```python
from build123d import *

# Parameters (mm, degrees)
SALIENTE_EXTRUIR1_DEPTH = 15
CROQUIS2_R              = 2.5
CORTAR_EXTRUIR1_DEPTH   = 3.5
CORTAR_EXTRUIR2_START   = -3.5
CROQUIS3_R              = 2.5
CORTAR_EXTRUIR2_DEPTH   = 3.5
CROQUIS4_R              = 2.5
CORTAR_EXTRUIR3_DEPTH   = 2
REDONDEO1_R             = 0.1
CROQUIS5_R              = 1.5
CORTAR_EXTRUIR4_DEPTH   = 26.421447638


with BuildPart() as part:
    # Croquis1 → Saliente-Extruir1 (new body)
    with BuildSketch(Plane.XY):
        with BuildLine():
            Line((-1.5, 11), (1.5, 11))
            ThreePointArc((1.5, 11), (4.328427125, 9.828427125), (5.5, 7))
            Line((5.5, 7), (5.5, -6))
            Line((5.5, -6), (11.5, -6))
            Line((11.5, -6), (11.5, -11))
            Line((11.5, -11), (5.5, -11))
            Line((5.5, -11), (-5.5, -11))
            Line((-5.5, -11), (-11.5, -11))
            Line((-11.5, -11), (-11.5, -6))
            Line((-11.5, -6), (-5.5, -6))
            Line((-5.5, -6), (-5.5, 7))
            ThreePointArc((-5.5, 7), (-4.328427125, 9.828427125), (-1.5, 11))
        make_face()
    extrude(amount=-SALIENTE_EXTRUIR1_DEPTH)

    # Croquis2 → Cortar-Extruir1 (cut)
    with BuildSketch(Plane(origin=(5.5, 0, 0), x_dir=(0, 0, -1), z_dir=(1, 0, 0))):
        with Locations(Location((7.5, 2.7, 0), (0, 0, 90))):
            Circle(CROQUIS2_R)
    extrude(amount=-CORTAR_EXTRUIR1_DEPTH, mode=Mode.SUBTRACT)

    # Croquis3 → Cortar-Extruir2 (cut)
    with BuildSketch(Plane.ZY.offset(5.5).offset(CORTAR_EXTRUIR2_START)):
        with Locations(Location((-7.5, 2.7, 0), (0, 0, 90))):
            Circle(CROQUIS3_R)
    extrude(amount=CORTAR_EXTRUIR2_DEPTH, mode=Mode.SUBTRACT)

    # Croquis4 → Cortar-Extruir3 (cut)
    with BuildSketch(Plane(origin=(0, -6, 0), x_dir=(1, 0, 0), z_dir=(0, 1, 0))):
        with Locations(Location((-8.5, 11, 0), (0, 0, 180))):
            Circle(CROQUIS4_R)
        with Locations(Location((-8.5, 4, 0), (0, 0, 180))):
            Circle(CROQUIS4_R)
        with Locations((8.5, 4)):
            Circle(CROQUIS4_R)
        with Locations((8.5, 11)):
            Circle(CROQUIS4_R)
    extrude(amount=-CORTAR_EXTRUIR3_DEPTH, mode=Mode.SUBTRACT)

    # Redondeo1
    redondeo1_edges = [part.edges().sort_by_distance(p)[0] for p in [
        (6, -6, -11),
        (6, -6, -4),
        (-6, -6, -4),
        (-6, -6, -11),
    ]]
    fillet(redondeo1_edges, radius=REDONDEO1_R)

    # Croquis5 → Cortar-Extruir4 (cut, through all)
    with BuildSketch(Plane(origin=(0, -6, 0), x_dir=(1, 0, 0), z_dir=(0, 1, 0))):
        with Locations(Location((-8.5, 11, 0), (0, 0, 180))):
            Circle(CROQUIS5_R)
        with Locations(Location((-8.5, 4, 0), (0, 0, 180))):
            Circle(CROQUIS5_R)
        with Locations((8.5, 4)):
            Circle(CROQUIS5_R)
        with Locations((8.5, 11)):
            Circle(CROQUIS5_R)
    extrude(amount=-CORTAR_EXTRUIR4_DEPTH, mode=Mode.SUBTRACT)


solid = part.part
```
Check sheet for the modelled part. Datum: model origin and axes. Units: mm. A direction names the side the tool comes from. Coordinates: 2 decimals unless noted, no trailing zeros. Loops run counter-clockwise (first coordinate to the right, second up) from the corner with the lowest first, then second, coordinate; pieces in that order, holes last.
1) Sectioned sample at B-B (x = 8.5). Record the boundary of the cut face in (y, z).
2) Gauge pin test, flat ends, axial feed: pin 1 (4 mm diameter, centred on x = 8.5, z = -10, fed in from +Y); pin 2 (4.5 mm diameter, centred on x = -8.5, z = -11, fed in from +Y); pin 3 (6.5 mm diameter, centred on x = 8, z = -7, fed in from +Y); pin 4 (3.5 mm diameter, centred on x = -8.5, z = -11, fed in from -Y). Record the tip position at first contact, or that the pin passes through.
3) Sectioned sample at A-A (z = -11). Count the separate pieces of the cut face and the enclosed holes in it, and give its area (3 significant figures).
4) Release check for a two-part mould opening along X. For faces 1 (the face through (-7.39, -9.48, -2.99)), 2 (the face through (0, -2, 0)), 3 (the face through (-2, 3, -8)), 4 (the face through (-10, -8, -5)) record: released by +X, released by -X, zero draft, split by the parting line, or undercut.
5) Access from +Z, -Z, +X, -X, +Y, -Y to the whole of each face (thin tool, end or side, straight path). Record for faces 5 (the face through (2, 3, -7)), 6 (the face through (8, -6, -7)), 7 (the face through (-10, -8, -12)).
6) Sectioned sample at C-C (z = -7.5). Record the boundary of the cut face in (x, y).
7) Sectioned sample at D-D (y = 1.75). Record the boundary of the cut face in (x, z).
8) Material ranges on probe 1 along Z at (x, y) = (-8.5, -9.95); probe 2 along Z at (x, y) = (8.5, -7.25); probe 3 along Z at (x, y) = (2.95, 2.7), recorded low to high.
Check sheet entries:
1. outline: (-11, -15) - (-6, -15) - (-6, -13.6) arc R0.1 ccw to (-6.1, -13.5) - (-8, -13.5) - (-8, -12.5) - (-11, -12.5) - close; (-11, -9.5) - (-8, -9.5) - (-8, -8.5) - (-6.1, -8.5) arc R0.1 ccw to (-6, -8.4) - (-6, -6.6) arc R0.1 ccw to (-6.1, -6.5) - (-8, -6.5) - (-8, -5.5) - (-11, -5.5) - close; (-11, -2.5) - (-8, -2.5) - (-8, -1.5) - (-6.1, -1.5) arc R0.1 ccw to (-6, -1.4) - (-6, 0) - (-11, 0) - close
2. pin 1: stops at y = -6
2. pin 2: stops at y = -8
2. pin 3: stops at y = 9.33
2. pin 4: stops at y = -11
3. separate pieces: 3
3. enclosed holes: 0
3. area: 257 mm2
4. face 1: undercut
4. face 2: zero draft
4. face 3: released by -X
4. face 4: undercut
5. face 5: +X
5. face 6: +Z, -Z, +X, +Y
5. face 7: +Y
6. outline: (-11.5, -11) - (11.5, -11) - (11.5, -6) - (5.5, -6) - (5.5, 0.2) - (2, 0.2) - (2, 5.2) - (5.5, 5.2) - (5.5, 7) arc R4 ccw to (1.5, 11) - (-1.5, 11) arc R4 ccw to (-5.5, 7) - (-5.5, 5.2) - (-2, 5.2) - (-2, 0.2) - (-5.5, 0.2) - (-5.5, -6) - (-11.5, -6) - close
7. outline: (-5.5, -15) - (5.5, -15) - (5.5, -9.81) - (2, -9.81) - (2, -5.19) - (5.5, -5.19) - (5.5, 0) - (-5.5, 0) - (-5.5, -5.19) - (-2, -5.19) - (-2, -9.81) - (-5.5, -9.81) - close
8. probe 1: z = -15 to -12.5, -9.5 to -5.5, -2.5 to 0
8. probe 2: z = -15 to -13.5, -8.5 to -6.5, -1.5 to 0
8. probe 3: z = -15 to -10, -5 to 0
